Design review of the part built by this model. Coordinates are the model's own, in mm. A direction names the side the tool comes from. Give positions to 0.01 mm unless a question says otherwise; leave off trailing zeros. Order: outer loops, then holes, each group sorted by start corner. A loop starts at its lowest first (then second) coordinate and runs counter-clockwise, first axis right, second up. Notation, with made-up numbers: M 10,54 L 59,54 A30 ccw 59,87 Z; hole C 3.5,3 d2. An arc over 180 degrees is marked long. Answer as a JSON object with one key per item and string values.
from build123d import *

# Parameters (mm, degrees)
F0_R            = 24.51608
F0_R_2          = 3.96875
F0_R_3          = 2.15265
F0_R_4          = 11.1125
F1_DEPTH        = 3.175
F3_DEPTH        = 3.175
F3_COPIES_COUNT = 4
F4_R            = 0.762


# Not quite as in the source:
# - a pattern or mirror of a feature is missing from the dataset's text; its kind, count and spacing are read off the source's solid


with BuildPart() as f1:
    # F0 (on Top) → F1 (new body)
    with BuildSketch(Plane.XY):
        Circle(F0_R)
        with Locations((-11.7865861589, -11.7865861589)):
            Circle(F0_R_2, mode=Mode.SUBTRACT)
        with Locations((11.7865861589, -11.7865861589)):
            Circle(F0_R_3, mode=Mode.SUBTRACT)
        with Locations((-11.7865861589, 11.7865861589)):
            Circle(F0_R_3, mode=Mode.SUBTRACT)
        Circle(F0_R_4, mode=Mode.SUBTRACT)
        with Locations((11.7865861589, 11.7865861589)):
            Circle(F0_R_2, mode=Mode.SUBTRACT)
    extrude(amount=F1_DEPTH)

    # F2 (on face) → F3 (cut, through all)
    with BuildSketch(Plane.XY.offset(3.175)):
        with BuildLine():
            ThreePointArc((-12.5005283394, 17.296776775), (-8.5209489043, 16.2818645023), (-6.3255746232, 12.8109235396))
            ThreePointArc((-6.3255746232, 12.8109235396), (0, 14.2875), (6.3255746232, 12.8109235396))
            ThreePointArc((6.3255746232, 12.8109235396), (8.5209489043, 16.2818645023), (12.5005283394, 17.296776775))
            ThreePointArc((12.5005283394, 17.296776775), (0, 21.34108), (-12.5005283394, 17.296776775))
        make_face()
    f3 = extrude(amount=-F3_DEPTH, mode=Mode.SUBTRACT)

    # F3_copies: F3 ×4 about axis
    f3_copies_axis = Axis((0, 0, 0), (0, 0, 1))
    for i in range(1, F3_COPIES_COUNT):
        add(f3.rotate(f3_copies_axis, i * 360 / F3_COPIES_COUNT), mode=Mode.SUBTRACT)

    # F4
    f4_edges = [f1.edges().sort_by_distance(p)[0] for p in [
        (-12.500528, 17.296777, 1.5875),
        (12.500528, 17.296777, 1.5875),
        (12.500528, -17.296777, 1.5875),
        (-12.500528, -17.296777, 1.5875),
        (17.296777, 12.500528, 1.5875),
        (17.296777, -12.500528, 1.5875),
        (-17.296777, -12.500528, 1.5875),
        (-17.296777, 12.500528, 1.5875),
    ]]
    fillet(f4_edges, radius=F4_R)


solid = f1.part
(1) Insertion check: pin 1 (10.5 mm diameter, centred on x = -11.79, y = -11.79, fed in from +Z) (3 decimals); pin 2 (18 mm diameter, centred on x = 0, y = 0, fed in from -Z). Each pin has a flat end and moves straight along its axis. Give the tip position at first contact, or say it passes through.
Checked values:
{"pin 1": "stops at z = 3.175", "pin 2": "passes through"}
(2) Tool access review of faces 1 (the cylindrical face through (-0.15, -21.34, 1.61)), 2 (the flat face through (11, -5, 3.175)): name each direction out of +Z, -Z, +X, -X, +Y, -Y from which nothing blocks a thin tool from reaching the whole face with its end or side.
Checked values:
{"face 1": "+Z, -Z", "face 2": "+Z, +X, -X, +Y, -Y"}
(3) Draft analysis for pull direction X (two halves, no side actions). For faces 3 (the flat face through (11, -5, 0)), 4 (the cylindrical face through (7.685, 15.535, 1.61)), state which applies: +X half, -X half, draft (parallel to the pull), parting line (faces both ways), or undercut.
Checked values:
{"face 3": "draft", "face 4": "undercut"}
(4) We need section C-C (z = 1.1). Count the separate pieces of the cut face and the enclosed holes in it, plus the area to 3 significant figures.
Checked values:
{"separate pieces": "1", "enclosed holes": "9", "area": "880 mm^2"}
(5) To check wall thickness, follow L1, parallel to Y at x = 0, z = 2.45; L2, parallel to Y at x = 7, z = 0.85; L3, parallel to X at y = -5, z = 0.55. State the ranges of each line that lie inside material, in increasing order. Write a range as from..to.
Checked values:
{"L1": "y = -24.52..-21.34, -14.29..-11.11, 11.11..14.29, 21.34..24.52", "L2": "y = -23.5..-20.16, -14.61..-8.63, 8.63..14.61, 20.16..23.5", "L3": "x = -24..-20.75, -13.38..-9.92, 9.92..13.38, 20.75..24"}
(6) We need section A-A (x = 0). Write out the cut boundary in (y, z) (1 decimal).
Checked values:
{"outline": "M -24.5,0 L -21.3,0 L -21.3,3.2 L -24.5,3.2 Z; M -14.3,0 L -11.1,0 L -11.1,3.2 L -14.3,3.2 Z; M 11.1,0 L 14.3,0 L 14.3,3.2 L 11.1,3.2 Z; M 21.3,0 L 24.5,0 L 24.5,3.2 L 21.3,3.2 Z"}
